For this review, take the finished solid that the model builds, in its own axes (mm). Coordinates: 2 decimals unless noted, no trailing zeros. Write each loop counter-clockwise with the first axis right and the second up, starting at its lowest first coordinate (ties: lowest second). Pieces come first, ordered by that corner, then holes. Notation, with made-up numbers: (-18, -34) -> (32, -34) arc R6 ccw to (32, -27) -> close; hole circle Ø5 at (-3.75, 63.5). An arc over 180 degrees is marked (long way). Put each result on its own line as item: value. Start each with the question number.
Item 1: Insertion check: P1, Ø0.8, axis at y = 4.5, z = 1, coming from the +X side. The pin has a flat end and moves straight along its axis. Give the tip position at first contact, or say it passes through.
Item 2: To check wall thickness, follow L1, parallel to Y at x = 50, z = 1; L2, parallel to Y at x = -65, z = 0.7; L3, parallel to X at y = 24.5, z = 1.3. State the ranges of each line that lie inside material, in increasing order.
Item 3: The part is to be moulded in two halves that separate along Y. For faces 1 (the cylindrical face through (-48.383, 34.33, 0.74)), 2 (the flat face through (-1, 1, 1.5)), 3 (the cylindrical face through (51.617, 34.33, 0.74)), say which applies: +Y half, -Y half, draft (parallel to the pull), parting line (faces both ways), or undercut.
Item 4: Consider section B-B on y = 55. Give the boundary of the cut face in (x, z), and give its area (4 significant figures).
Item 5: Consider section C-C on z = 1.1. Give the number of separate pieces and of enclosed holes in the cut face, and give its area (3 significant figures).
Item 6: Consider section A-A on x = -50. Give the boundary of the cut face in (y, z), and give its area (4 significant figures).
Item 7: Consider section D-D on x = 65. Give the boundary of the cut face in (y, z).
```python
from build123d import *

# Parameters (mm, degrees)
SKETCH_1_W          = 140
SKETCH_1_H          = 120
SKETCH_1_R          = 2.25
SKETCH_1_R_2        = 1.75
EXTRUDE_1_DEPTH     = 1.5
SKETCH_2_W          = 21.124168751
SKETCH_2_H          = 70
CUT_EXTRUDE_1_DEPTH = 10


with BuildPart() as part:
    # Эскиз1 → Вытянуть1 (new body)
    with BuildSketch(Plane.XY):
        Rectangle(SKETCH_1_W, SKETCH_1_H)
        with Locations((-65, 55)):
            Circle(SKETCH_1_R, mode=Mode.SUBTRACT)
        with Locations(Location((-65, -55, 0), (0, 0, 180))):
            Circle(SKETCH_1_R, mode=Mode.SUBTRACT)
        with Locations((65, -55)):
            Circle(SKETCH_1_R, mode=Mode.SUBTRACT)
        with Locations(Location((65, 55, 0), (0, 0, 180))):
            Circle(SKETCH_1_R, mode=Mode.SUBTRACT)
        with Locations((-50, 35)):
            Circle(SKETCH_1_R_2, mode=Mode.SUBTRACT)
        with Locations(Location((-50, -35, 0), (0, 0, 180))):
            Circle(SKETCH_1_R_2, mode=Mode.SUBTRACT)
        with Locations((50, 35)):
            Circle(SKETCH_1_R_2, mode=Mode.SUBTRACT)
        with Locations(Location((50, -35, 0), (0, 0, 180))):
            Circle(SKETCH_1_R_2, mode=Mode.SUBTRACT)
    extrude(amount=EXTRUDE_1_DEPTH)

    # Эскиз2 → Вырез-Вытянуть1 (cut)
    with BuildSketch(Plane.XY.offset(1.5)):
        with Locations((68.562084376, 0)):
            Rectangle(SKETCH_2_W, SKETCH_2_H)
    extrude(amount=-CUT_EXTRUDE_1_DEPTH, mode=Mode.SUBTRACT)


solid = part.part
```
Return value:
1. P1: x = 58
2. L1: -60 to -36.75, -33.25 to 33.25, 36.75 to 60
2. L2: -60 to -57.25, -52.75 to 52.75, 57.25 to 60
2. L3: -70 to 58
3. face 1: undercut
3. face 2: draft
3. face 3: undercut
4. outline: (-70, 0) -> (-67.25, 0) -> (-67.25, 1.5) -> (-70, 1.5) -> close; (-62.75, 0) -> (62.75, 0) -> (62.75, 1.5) -> (-62.75, 1.5) -> close; (67.25, 0) -> (70, 0) -> (70, 1.5) -> (67.25, 1.5) -> close
4. area: 196.5 mm^2
5. separate pieces: 1
5. enclosed holes: 8
5. area: 15,900 mm^2
6. outline: (-60, 0) -> (-36.75, 0) -> (-36.75, 1.5) -> (-60, 1.5) -> close; (-33.25, 0) -> (33.25, 0) -> (33.25, 1.5) -> (-33.25, 1.5) -> close; (36.75, 0) -> (60, 0) -> (60, 1.5) -> (36.75, 1.5) -> close
6. area: 169.5 mm^2
7. outline: (-60, 0) -> (-57.25, 0) -> (-57.25, 1.5) -> (-60, 1.5) -> close; (-52.75, 0) -> (-35, 0) -> (-35, 1.5) -> (-52.75, 1.5) -> close; (35, 0) -> (52.75, 0) -> (52.75, 1.5) -> (35, 1.5) -> close; (57.25, 0) -> (60, 0) -> (60, 1.5) -> (57.25, 1.5) -> close
